```python
from build123d import *

# Parameters (mm, degrees)
SKETCH_1_W             = 33
SKETCH_1_H             = 14.3
SKETCH_1_W_2           = 29
SKETCH_1_H_2           = 10.3
EXTRUDE_2_DEPTH        = 36
SKETCH_2_W             = 33
SKETCH_2_H             = 14.3
SKETCH_2_RX            = 14.5
SKETCH_2_RY            = 5.15
EXTRUDE_3_DEPTH        = 3
PATTERN_LINEAR_1_COUNT = 2
PATTERN_LINEAR_1_PITCH = 13.5


with BuildPart() as part:
    # 草图1 → 凸台-拉伸2 (new body)
    with BuildSketch(Plane(origin=(0, 0, 0), x_dir=(1, 0, 0), z_dir=(0, 1, 0))):
        Rectangle(SKETCH_1_W, SKETCH_1_H)
        Rectangle(SKETCH_1_W_2, SKETCH_1_H_2, mode=Mode.SUBTRACT)
    extrude_2 = extrude(amount=EXTRUDE_2_DEPTH)

    # 草图2 → 凸台-拉伸3 (add)
    with BuildSketch(Plane(origin=(0, 36, 0), x_dir=(1, 0, 0), z_dir=(0, 1, 0))):
        Rectangle(SKETCH_2_W, SKETCH_2_H)
        with Locations(Location((0, 0), (0, 0, 0))):
            Ellipse(SKETCH_2_RX, SKETCH_2_RY, mode=Mode.SUBTRACT)
    extrude_3 = extrude(amount=EXTRUDE_3_DEPTH)

    # 阵列(线性)1: 凸台-拉伸2, 凸台-拉伸3 ×2
    with Locations(*[(0, 0, i * PATTERN_LINEAR_1_PITCH) for i in range(1, PATTERN_LINEAR_1_COUNT)]):
        add(extrude_2)
        add(extrude_3)


solid = part.part
```
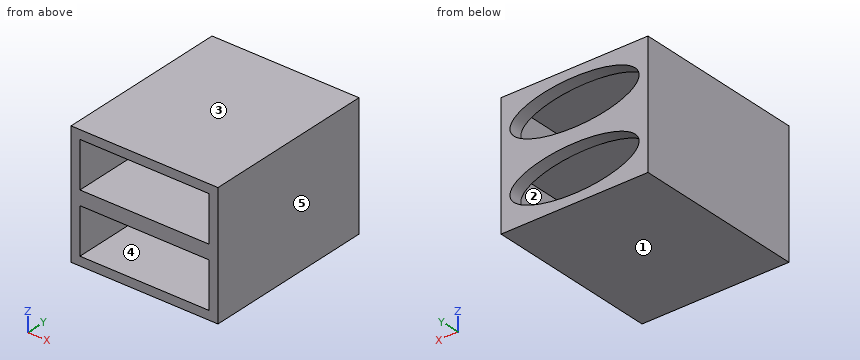
The listing builds one solid part. Answer for the finished solid, in the listing's coordinates (mm). Face numbers are marked on the shaded views. A direction names the side the tool comes from. Round coordinates to 2 decimals unless told otherwise and drop trailing zeros. Loops run counter-clockwise (first coordinate to the right, second up) from the corner with the lowest first, then second, coordinate; pieces in that order, holes last.
Q1. Section A-A, the plane y = 23.5 is taken. Determine the outline of the cut face in (x, z), then the cut area to 3 significant figures.
Q2. Which of the six approach directions +Z, -Z, +X, -X, +Y, -Y give full straight-line access (tool end or side, diameter ignored) to the marked faces 1 and 2?
Q3. Given pin 1 Ø1.5 at (x, z) = (5.5, 16) entering from -Y; pin 2 Ø2.5 at (x, z) = (-10, 11) entering from -Y, each flat-ended and moving along its own axis, determine where each tip first touches the part or whether it passes through.
Q4. Section B-B, the plane x = 8.5 is taken. Count the separate pieces of the cut face and the enclosed holes in it, then the cut area to 3 significant figures.
Q5. For a pull along Z with two mould halves and no side action, classify the marked faces 3, 4 and 5 as released by +Z, released by -Z, zero draft, split by the parting line, or undercut.
Q6. Find the intervals of material crossed by line 1 (Z direction, x = 8, y = 20); line 2 (X direction, y = 34.5, z = 18.5); line 3 (Z direction, x = 12.5, y = 37), in increasing order.
Completed:
1. outline: (-16.5, -7.15) - (16.5, -7.15) - (16.5, 20.65) - (-16.5, 20.65) - close; hole (-14.5, -5.15) - (14.5, -5.15) - (14.5, 5.15) - (-14.5, 5.15) - close; hole (-14.5, 8.35) - (14.5, 8.35) - (14.5, 18.65) - (-14.5, 18.65) - close
1. area: 320 mm2
2. face 1: -Z, +X, -X, +Y, -Y
2. face 2: -Y
3. pin 1: passes through
3. pin 2: stops at y = 36
4. separate pieces: 3
4. enclosed holes: 0
4. area: 293 mm2
5. face 3: released by +Z
5. face 4: undercut
5. face 5: zero draft
6. line 1: z = -7.15 to -5.15, 5.15 to 8.35, 18.65 to 20.65
6. line 2: x = -16.5 to -14.5, 14.5 to 16.5
6. line 3: z = -7.15 to -2.61, 2.61 to 10.89, 16.11 to 20.65
